from build123d import *

# Parameters (mm, degrees)
SKETCH_W            = 77.5
SKETCH_H            = 52.5
SKETCH_R            = 1.6
PAD_DEPTH           = 1.6
SKETCH004_W         = 16.5
SKETCH004_H         = 22.5
PAD004_DEPTH        = 19
LINEARPATTERN_COUNT = 4
LINEARPATTERN_PITCH = 19.333333


with BuildPart() as part:
    # Sketch → Pad (new body)
    with BuildSketch(Plane.XY):
        Rectangle(SKETCH_W, SKETCH_H)
        with Locations((-35.25, 22.65)):
            Circle(SKETCH_R, mode=Mode.SUBTRACT)
        with Locations((-35.25, -22.65)):
            Circle(SKETCH_R, mode=Mode.SUBTRACT)
        with Locations((35.25, 22.65)):
            Circle(SKETCH_R, mode=Mode.SUBTRACT)
        with Locations((35.25, -22.65)):
            Circle(SKETCH_R, mode=Mode.SUBTRACT)
    extrude(amount=PAD_DEPTH)

    # Sketch004 (on Face10 of Pad) → Pad004 (join)
    with BuildSketch(Plane.XY.offset(1.6)):
        with Locations((-29.499962, 4.46239)):
            Rectangle(SKETCH004_W, SKETCH004_H)
    pad004 = extrude(amount=PAD004_DEPTH)

    # LinearPattern: Pad004 ×4
    with Locations(*[(i * LINEARPATTERN_PITCH, 0, 0) for i in range(1, LINEARPATTERN_COUNT)]):
        add(pad004)


solid = part.part
Work out the finished part from the listing and answer in its coordinate system (mm). A direction names the side the tool comes from. Coordinates: 2 decimals unless noted, no trailing zeros. Write each loop counter-clockwise with the first axis right and the second up, starting at its lowest first coordinate (ties: lowest second). Pieces come first, ordered by that corner, then holes.
1. The part is cut by section A-A, the plane z = 16.5. Write down the section's boundary in (x, y), and give its area (4 significant figures).
Results list:
outline: (-37.75, -6.79) - (-21.25, -6.79) - (-21.25, 15.71) - (-37.75, 15.71) - close; (-18.42, -6.79) - (-1.92, -6.79) - (-1.92, 15.71) - (-18.42, 15.71) - close; (0.92, -6.79) - (17.42, -6.79) - (17.42, 15.71) - (0.92, 15.71) - close; (20.25, -6.79) - (36.75, -6.79) - (36.75, 15.71) - (20.25, 15.71) - close
area: 1,485 mm2
2. The part is cut by section D-D, the plane x = -6.5. Write down the section's boundary in (y, z).
Results list:
outline: (-26.25, 0) - (26.25, 0) - (26.25, 1.6) - (15.71, 1.6) - (15.71, 20.6) - (-6.79, 20.6) - (-6.79, 1.6) - (-26.25, 1.6) - close
3. For faces 4 (the flat face through (-1.917, 4, 11)), 5 (the flat face through (9, -6.788, 11)), 6 (the flat face through (-10, 15.712, 11)), 7 (the cylindrical face through (33.65, -22.58, 0.79)), determine the directions among +Z, -Z, +X, -X, +Y, -Y from which every point of the face is accessible in a straight line to the end or side of a thin tool.
Results list:
face 4: +Z, +Y, -Y
face 5: +Z, +X, -X, -Y
face 6: +Z, +X, -X, +Y
face 7: +Z, -Z
4. The part is cut by section C-C, the plane y = 22.65. Write down the section's boundary in (x, z).
Results list:
outline: (-38.75, 0) - (-36.85, 0) - (-36.85, 1.6) - (-38.75, 1.6) - close; (-33.65, 0) - (33.65, 0) - (33.65, 1.6) - (-33.65, 1.6) - close; (36.85, 0) - (38.75, 0) - (38.75, 1.6) - (36.85, 1.6) - close
5. For a pull along X with two mould halves and no side action, classify faces 1 (the cylindrical face through (33.98, 21.68, 0.79)), 2 (the flat face through (-38.75, 0, 1)), 3 (the flat face through (9, 5, 20.6)) as +X half, -X half, draft (parallel to the pull), parting line (faces both ways), or undercut.
Results list:
face 1: undercut
face 2: -X half
face 3: draft
6. Flat-ended cylindrical pins translate along their axes: pin 1 (10 mm diameter, centred on x = 19.5, z = 7, fed in from +Y); pin 2 (3.5 mm diameter, centred on x = -35.25, y = -22.65, fed in from +Z); pin 3 (8 mm diameter, centred on y = 12, z = 14, fed in from -X); pin 4 (1.9 mm diameter, centred on x = 35.25, y = 22.65, fed in from -Z). Find the tip coordinate at first contact, or state that the pin passes through.
Results list:
pin 1: stops at y = 15.71
pin 2: stops at z = 1.6
pin 3: stops at x = -37.75
pin 4: passes through
7. The part is cut by section B-B, the plane x = 35.25. Write down the section's boundary in (y, z).
Results list:
outline: (-26.25, 0) - (-24.25, 0) - (-24.25, 1.6) - (-26.25, 1.6) - close; (-21.05, 0) - (21.05, 0) - (21.05, 1.6) - (15.71, 1.6) - (15.71, 20.6) - (-6.79, 20.6) - (-6.79, 1.6) - (-21.05, 1.6) - close; (24.25, 0) - (26.25, 0) - (26.25, 1.6) - (24.25, 1.6) - close
8. Consider line 1 along Y through (x, z) = (-35.25, 1.15); line 2 along X through (y, z) = (8, 5.75); line 3 along Y through (x, z) = (-28, 18). Determine where each line is inside the solid, lowest interval first.
Results list:
line 1: y = -26.25 to -24.25, -21.05 to 21.05, 24.25 to 26.25
line 2: x = -37.75 to -21.25, -18.42 to -1.92, 0.92 to 17.42, 20.25 to 36.75
line 3: y = -6.79 to 15.71
